Can you work these out from the model? Positions are in its coordinate system, mm. A direction names the side the tool comes from. Round coordinates to 2 decimals unless told otherwise and drop trailing zeros. Loops run counter-clockwise (first coordinate to the right, second up) from the corner with the lowest first, then second, coordinate; pieces in that order, holes last. Notation, with made-up numbers: M 33,80.25 L 90,80.25 A18 cw 90,109.25 Z; hole C 74.25,61 d2. An arc over 180 degrees is marked long. Return JSON: item names as keys, results as strings.
```python
from build123d import *

# Parameters (mm, degrees)
F0_W     = 254
F0_H     = 19.05
F1_DEPTH = 12.7
F2_R     = 3.1115
F3_DEPTH = 12.7
F4_W     = 9.525
F4_H     = 9.525
F4_R     = 3.1115
F5_DEPTH = 12.7
F6_DEPTH = 25.4


# Not quite as in the source:
# - a feature names something its author has since deleted; it is built from what else it names


with BuildPart() as f1:
    # F0 (on Front) → F1 (new body)
    with BuildSketch(Plane.XZ):
        Rectangle(F0_W, F0_H)
    extrude(amount=F1_DEPTH)

    # F2 (on face) → F3 (join)
    with BuildSketch(Plane.XZ.offset(12.7)):
        Circle(F2_R)
    extrude(amount=F3_DEPTH)

    # F4 (on face) → F5 (join)
    with BuildSketch(Plane(origin=(0, 0, 0), x_dir=(-1, 0, 0), z_dir=(0, 1, 0))):
        with Locations((-114.3, 0)):
            Rectangle(F4_W, F4_H)
        with Locations((-85.725, 0)):
            Circle(F4_R)
        with Locations((-57.15, 0)):
            Rectangle(F4_W, F4_H)
        with Locations((-28.575, 0)):
            Circle(F4_R)
        with Locations((28.575, 0)):
            Circle(F4_R)
        with Locations((57.15, 0)):
            Rectangle(F4_W, F4_H)
        with Locations((85.725, 0)):
            Circle(F4_R)
        with Locations((114.3, 0)):
            Rectangle(F4_W, F4_H)
    extrude(amount=F5_DEPTH)

    # F6 (cut): faces of the model
    f6_faces = [f1.faces().sort_by_distance(p)[0] for p in [
        (114.3, 12.7, 0),
        (57.15, 12.7, 0),
        (-57.15, 12.7, 0),
        (-114.3, 12.7, 0),
    ]]
    extrude(f6_faces, amount=-F6_DEPTH, mode=Mode.SUBTRACT)


solid = f1.part
```
Q1. On a 3-axis mill with a long thin cutter (end or side, diameter ignored), from which of +Z, -Z, +X, -X, +Y, -Y can I reach the whole of each face in a straight line? I mean faces 5 (the cylindrical face through (25.7, 6.26, -1.19)), 6 (the cylindrical face through (-0.67, -18.96, -3.04)), 7 (the flat face through (-2, -6, -9.525)), 8 (the flat face through (109.538, -6, 0)). Say none if no direction works.
Results:
{"face 5": "+Y", "face 6": "-Y", "face 7": "-Z, +X, -X, +Y, -Y", "face 8": "+Y, -Y"}
Q2. Suppose I cut it at B-B, the plane x = 0. Please give me the cut outline in (y, z) (1 decimal).
Results:
{"outline": "M -25.4,-3.1 L -12.7,-3.1 L -12.7,-9.5 L 0,-9.5 L 0,9.5 L -12.7,9.5 L -12.7,3.1 L -25.4,3.1 Z"}
Q3. Thinking about a two-plate mould opening in Z: for faces 1 (the flat face through (57, -6, -4.762)), 2 (the flat face through (114, -6, 4.762)), 3 (the cylindrical face through (88.194, 6.261, -1.893)), 4 (the flat face through (-2, 0, 0)), which applies, pulls with the +Z half, pulls with the -Z half, needs draft (parallel to the pull), parting line crosses it, or undercut?
Results:
{"face 1": "undercut", "face 2": "undercut", "face 3": "parting line crosses it", "face 4": "needs draft"}
Q4. Suppose I cut it at D-D, the plane y = 4. Please give me the cut outline in (x, z) (1 decimal).
Results:
{"outline": "C -85.7,0 d6.2; C -28.6,0 d6.2; C 28.6,0 d6.2; C 85.7,0 d6.2"}
Q5. Suppose I cut it at C-C, the plane z = 0. State how many separate pieces and enclosed holes the cut face has, plus the area to 3 significant figures.
Results:
{"separate pieces": "5", "enclosed holes": "0", "area": "3,140 mm2"}
Q6. If I drill on line 1 along X through (y, z) = (-8, 3.5); line 2 along Y through (x, z) = (90.5, -1.5); line 3 along Z through (x, y) = (114.5, -11) (1 decimal), over which ranges is the centre line in solid material (lowest first)?
Results:
{"line 1": "x = -127 to -119.06, -109.54 to -61.91, -52.39 to 52.39, 61.91 to 109.54, 119.06 to 127", "line 2": "y = -12.7 to 0", "line 3": "z = -9.5 to -4.8, 4.8 to 9.5"}
Q7. Suppose I cut it at A-A, the plane y = -6. Please give me the cut outline in (x, z) (1 decimal).
Results:
{"outline": "M -127,-9.5 L 127,-9.5 L 127,9.5 L -127,9.5 Z; hole M -119.1,-4.8 L -109.5,-4.8 L -109.5,4.8 L -119.1,4.8 Z; hole M -61.9,-4.8 L -52.4,-4.8 L -52.4,4.8 L -61.9,4.8 Z; hole M 52.4,-4.8 L 61.9,-4.8 L 61.9,4.8 L 52.4,4.8 Z; hole M 109.5,-4.8 L 119.1,-4.8 L 119.1,4.8 L 109.5,4.8 Z"}
Q8. I'm going to push flat-ended pins straight in: pin 1 Ø1 at (x, z) = (50, -7.5) entering from +Y; pin 2 Ø3 at (x, z) = (5, -2.5) entering from -Y; pin 3 Ø5 at (x, y) = (-1.5, -19.5) entering from +Z. Where does each tip first touch, or does it pass through?
Results:
{"pin 1": "stops at y = 0", "pin 2": "stops at y = -12.7", "pin 3": "stops at z = 3.11"}
